from build123d import *

# Parameters (mm, degrees)
F1_DEPTH    = 15
F2_R        = 8.5
F2_W        = 6
F2_H        = 15
F3_DEPTH    = 25
F4_SIZE2    = 19
F4_SIZE     = 1
F5_R        = 2
F6_R        = 5
F7_T1_DEPTH = 15
F7_T4_ANGLE = 90
F7_T6_ANGLE = 90


# Not quite as in the source:
# - a fillet or chamfer that OpenCascade refuses, or shapes differently, is made with other operations: its cross-section is extruded or revolved along the edge and cut away or added


with BuildPart() as f1:
    # F0 (on Top) → F1 (new body)
    with BuildSketch(Plane.XY):
        with BuildLine():
            ThreePointArc((-21, 0), (-14.8492424049, -14.8492424049), (0, -21))
            Line((0, -21), (0, -15))
            ThreePointArc((0, -15), (-10.6066017178, -10.6066017178), (-15, 0))
            Line((-15, 0), (-21, 0))
        make_face()
        Polygon((0, -15), (0, -21), (6, -21), (6, 19), (0, 19), (0, 0), align=None)
    extrude(amount=F1_DEPTH)

    # F2 (on face) → F3 (join)
    with BuildSketch(Plane(origin=(0, 19, 0), x_dir=(-1, 0, 0), z_dir=(0, 1, 0))):
        with Locations((-3, 7.5)):
            Circle(F2_R)
        with Locations((-3, 7.5)):
            Rectangle(F2_W, F2_H, mode=Mode.SUBTRACT)
        with Locations((-3, 7.5)):
            Rectangle(F2_W, F2_H)
    extrude(amount=F3_DEPTH)

    # F4
    f4_edges = [f1.edges().sort_by_distance(p)[0] for p in [
        (11.5, 44, 7.5),
    ]]
    f4_side = f1.faces().sort_by_distance((3, 44, 7.5))[0]
    chamfer(f4_edges, length=F4_SIZE, length2=F4_SIZE2, reference=f4_side)

    # F5
    f5_edges = [f1.edges().sort_by_distance(p)[0] for p in [
        (6, -1, 15),
        (-14.849242, -14.849242, 15),
        (3, -21, 0),
        (-14.849242, -14.849242, 0),
        (6, -1, 0),
    ]]
    fillet(f5_edges, radius=F5_R)

    # F6
    f6_edges = [f1.edges().sort_by_distance(p)[0] for p in [
        (0, -15, 7.5),
    ]]
    fillet(f6_edges, radius=F6_R)

    # F7: fillet of radius 5 on 1 edges, made by hand

    # F7_s2 → F7_t1 (cut)
    with BuildSketch(Plane.XY):
        with BuildLine():
            ThreePointArc((6, -16), (4.5355339059, -19.5355339059), (1, -21))
            Line((1, -21), (6, -21))
            Line((6, -21), (6, -16))
        make_face()
    extrude(amount=F7_T1_DEPTH, mode=Mode.SUBTRACT)

    # F7_s3 → F7_t4 (revolve, cut)
    with BuildSketch(Plane.XZ.offset(16)):
        with BuildLine():
            ThreePointArc((4, 0), (5.4142135624, 0.5857864376), (6, 2))
            Line((6, 2), (6, 0))
            Line((6, 0), (4, 0))
        make_face()
    revolve(axis=Axis((1, -16, 0), (0, 0, -1)), revolution_arc=F7_T4_ANGLE, mode=Mode.SUBTRACT)

    # F7_s5 → F7_t6 (revolve, cut)
    with BuildSketch(Plane.YZ.offset(1)):
        with BuildLine():
            ThreePointArc((-19, 15), (-20.4142135624, 14.4142135624), (-21, 13))
            Line((-21, 13), (-21, 15))
            Line((-21, 15), (-19, 15))
        make_face()
    revolve(axis=Axis((1, -16, 15), (0, 0, 1)), revolution_arc=F7_T6_ANGLE, mode=Mode.SUBTRACT)


solid = f1.part
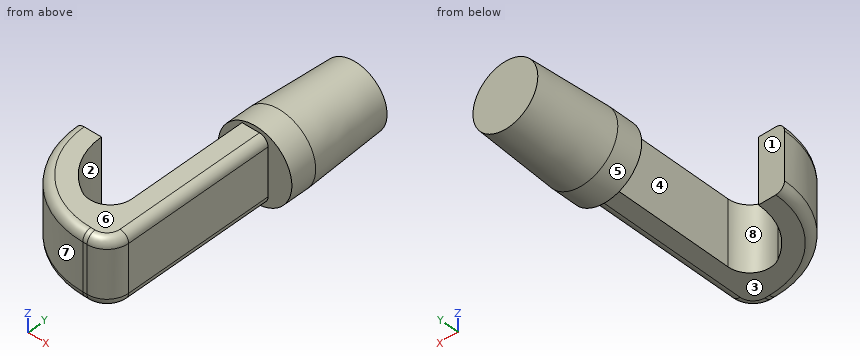
Build history of the part. All positions in model axes, mm. Face numbers are marked on the shaded views. A direction names the side the tool comes from. Round coordinates to 2 decimals unless told otherwise and drop trailing zeros. Write each loop counter-clockwise with the first axis right and the second up, starting at its lowest first coordinate (ties: lowest second). Pieces come first, ordered by that corner, then holes. Notation, with made-up numbers: (64.5, 38.25) - (77.5, 38.25) arc R5 cw to (77.5, 45.25) - close; hole circle Ø5 at (25.25, 71). An arc over 180 degrees is marked (long way). One line per question, with ' | ' between items.
1. Drop flat-ended pins along their axis: pin 1 Ø1.8 at (x, z) = (-18.5, 5.5) entering from +Y; pin 2 Ø3 at (y, z) = (10, 7) entering from -X; pin 3 Ø4 at (y, z) = (-11.5, 9.5) entering from -X. Give the stop position or say it passes through.
Results are:
pin 1: y = 0 | pin 2: x = 0 | pin 3: x = -18.73
2. Band-saw the part on A-A, the plane z = 7.5. Write the cut outline in (x, y).
Results are:
outline: (-21, 0) arc R21 ccw to (0, -21) - (1, -21) arc R5 ccw to (6, -16) - (6, 19) - (11.5, 19) - (11.5, 25) - (10.5, 44) - (-4.5, 44) - (-5.5, 25) - (-5.5, 19) - (0, 19) - (0, -8.66) arc R5 cw to (-7.5, -12.99) arc R15 cw to (-15, 0) - close
3. Band-saw the part on B-B, the plane y = 15. Write the cut outline in (x, z).
Results are:
outline: (0, 0) - (4, 0) arc R2 ccw to (6, 2) - (6, 13) arc R2 ccw to (4, 15) - (0, 15) - close
4. Mould opens along Y. For the marked faces 6, 7 and 8 say: released by +Y, released by -Y, zero draft, split by the parting line, or undercut.
Results are:
face 6: zero draft | face 7: released by -Y | face 8: undercut
5. Tool access for the marked faces 1, 2, 3, 4 and 5: list every direction of +Z, -Z, +X, -X, +Y, -Y with a clear straight run to the whole face (end or side of a thin tool).
Results are:
face 1: +Z, -Z, -X, +Y | face 2: +Z, -Z, +Y | face 3: -Z, +X, -X, -Y | face 4: +Z, -Z | face 5: +Y
6. Drill centre lines: line 1 along X through (y, z) = (3, 1.75); line 2 along Z through (x, y) = (-6, -18); line 3 along Y through (x, z) = (-16.5, 4). Where is each one in solid material? Low to high. Write a range as from..to.
Results are:
line 1: 0..5.98 | line 2: 0..15 | line 3: -12.99..0
